from build123d import *

# Parameters (mm, degrees)
SKETCH1_W               = 184
SKETCH1_H               = 15
BOSS_EXTRUDE1_DEPTH     = 7.25
CUT_EXTRUDE1_START      = -7.25
SKETCH1_6_W             = 184
SKETCH1_6_H             = 11
CUT_EXTRUDE1_DEPTH      = 3.5
CUT_EXTRUDE2_DEPTH      = 93.589483744
CUT_EXTRUDE2_DEPTH_BACK = 93.589483744
SKETCH2_R               = 3.5
SKETCH2_R_2             = 1.7
CHAMFER1_SIZE           = 0.4


with BuildPart() as part:
    # Sketch1 → Boss-Extrude1 (new body)
    with BuildSketch(Plane.XY):
        Rectangle(SKETCH1_W, SKETCH1_H)
    extrude(amount=-BOSS_EXTRUDE1_DEPTH)

    # Sketch1<6> → Cut-Extrude1 (cut)
    with BuildSketch(Plane.XY.offset(CUT_EXTRUDE1_START)):
        with Locations((0, -2)):
            Rectangle(SKETCH1_6_W, SKETCH1_6_H)
    extrude(amount=CUT_EXTRUDE1_DEPTH, mode=Mode.SUBTRACT)

    # Sketch2 → Cut-Extrude2 (cut, two sides: drawn at the far end of the back side and taken through both)
    with BuildSketch(Plane.XY.offset(-CUT_EXTRUDE2_DEPTH_BACK)):
        with Locations((-52.5, 0)):
            Circle(SKETCH2_R)
        with Locations((-36.25, 0)):
            Circle(SKETCH2_R_2)
        with Locations((-10.5, 0)):
            Circle(SKETCH2_R)
        Circle(SKETCH2_R_2)
        with Locations((10.5, 0)):
            Circle(SKETCH2_R)
        with Locations((36.25, 0)):
            Circle(SKETCH2_R_2)
        with Locations((52.5, 0)):
            Circle(SKETCH2_R)
        with Locations((-82.27, 0)):
            Circle(SKETCH2_R)
        with Locations((82.27, 0)):
            Circle(SKETCH2_R)
    extrude(amount=CUT_EXTRUDE2_DEPTH + CUT_EXTRUDE2_DEPTH_BACK, mode=Mode.SUBTRACT)

    # Chamfer1
    chamfer1_edges = [part.edges().sort_by_distance(p)[0] for p in [
        (-37.95, 0, 0),
        (-14, 0, 0),
        (-1.7, 0, 0),
        (7, 0, 0),
        (0, -7.5, 0),
        (78.77, 0, 0),
        (-92, 0, 0),
        (-85.77, 0, 0),
        (49, 0, 0),
        (34.55, 0, 0),
        (0, 7.5, 0),
        (-56, 0, 0),
        (92, 0, 0),
    ]]
    chamfer(chamfer1_edges, length=CHAMFER1_SIZE)


solid = part.part
Work out the finished part from the listing and answer in its coordinate system (mm). A direction names the side the tool comes from. Coordinates: 2 decimals unless noted, no trailing zeros. Write each loop counter-clockwise with the first axis right and the second up, starting at its lowest first coordinate (ties: lowest second). Pieces come first, ordered by that corner, then holes. Notation, with made-up numbers: (53, 72.5) - (58, 72.5) arc R7 ccw to (58, 76.5) - close; hole circle Ø5 at (69.5, 8). An arc over 180 degrees is marked (long way). One line per question, with ' | ' between items.
1) The mould has two halves that part along X. Classify faces 3 (the face through (92, 2, -2)), 4 (the face through (-56, 0, -2)), 5 (the face through (-1, 3.5, -6)), 6 (the face through (49, 0, -2)): +X half, -X half, draft (parallel to the pull), parting line (faces both ways), or undercut.
Checks:
face 3: +X half | face 4: undercut | face 5: draft | face 6: undercut
2) Find section A-A, the plane x = -36.25. Determine the outline of the cut face in (y, z), and give its area (3 significant figures).
Checks:
outline: (-7.5, -3.75) - (-1.7, -3.75) - (-1.7, -0.4) - (-2.1, 0) - (-7.1, 0) - (-7.5, -0.4) - close; (1.7, -3.75) - (3.5, -3.75) - (3.5, -7.25) - (7.5, -7.25) - (7.5, -0.4) - (7.1, 0) - (2.1, 0) - (1.7, -0.4) - close | area: 57.2 mm2
3) Find section C-C, the plane x = 76.5. Determine the outline of the cut face in (y, z).
Checks:
outline: (-7.5, -3.75) - (3.5, -3.75) - (3.5, -7.25) - (7.5, -7.25) - (7.5, -0.4) - (7.1, 0) - (-7.1, 0) - (-7.5, -0.4) - close
4) For faces 1 (the face through (-1, 7.5, -4)), 2 (the face through (-1, -2, -3.75)), determine the directions among +Z, -Z, +X, -X, +Y, -Y from which every point of the face is accessible in a straight line to the end or side of a thin tool.
Checks:
face 1: +Z, -Z, +X, -X, +Y | face 2: -Z, +X, -X, -Y
5) Consider probe 1 along Y at (x, z) = (-52.5, -1.6); probe 2 along Z at (x, y) = (-67, 2.5); probe 3 along Y at (x, z) = (-35, -5). Determine where each line is inside the solid, lowest interval first. Write a range as [from, to].
Checks:
probe 1: [-7.5, -3.5], [3.5, 7.5] | probe 2: [-3.75, 0] | probe 3: [3.5, 7.5]
6) Find section B-B, the plane y = 0. Give the number of separate pieces and of enclosed holes in the cut face, and give its area (3 significant figures).
Checks:
separate pieces: 10 | enclosed holes: 0 | area: 493 mm2
7) Flat-ended cylindrical pins translate along their axes: P1, Ø4.5, axis at x = 0, y = 0, coming from the -Z side; P2, Ø9, axis at x = 82.27, y = 0, coming from the -Z side; P3, Ø1, axis at x = -10.5, z = -6, coming from the -Y side. Find the tip coordinate at first contact, or state that the pin passes through.
Checks:
P1: z = -3.75 | P2: z = -7.25 | P3: y = 3.5
